Source: CAD feature listing. Evaluate the final solid. Frame: model axes, mm. A direction names the side the tool comes from. Round coordinates to 2 decimals unless told otherwise and drop trailing zeros. Write each loop counter-clockwise with the first axis right and the second up, starting at its lowest first coordinate (ties: lowest second). Pieces come first, ordered by that corner, then holes.
from build123d import *

# Parameters (mm, degrees)
SKETCH1_W          = 98.9
SKETCH1_H          = 124.45
BODY_DEPTH         = 22.55
SKETCH4_W          = 7
SKETCH4_H          = 3
SKETCH4_W_2        = 3
SKETCH4_H_2        = 7
CUT_EXTRUDE1_DEPTH = 63
SKETCH5_W          = 8.299397568
SKETCH5_H          = 10.9
CUT_EXTRUDE2_DEPTH = 63
SKETCH6_W          = 98.9
SKETCH6_H          = 68.5
CUT_EXTRUDE3_DEPTH = 63
SKETCH7_W          = 22.55
SKETCH7_H          = 1.441759006
CUT_EXTRUDE4_DEPTH = 63
SKETCH8_W          = 35
SKETCH8_H          = 13.1
CUT_EXTRUDE5_DEPTH = 23.55
SKETCH9_R          = 1.25
CUT_EXTRUDE6_DEPTH = 10
SKETCH10_R         = 1.25
CUT_EXTRUDE7_DEPTH = 5
CIRPATTERN1_COUNT  = 4


with BuildPart() as part:
    # Sketch1 → body (new body)
    with BuildSketch(Plane.XY):
        Rectangle(SKETCH1_W, SKETCH1_H)
    extrude(amount=BODY_DEPTH)

    # Sketch4 → Cut-Extrude1 (cut)
    with BuildSketch(Plane(origin=(0, 0, 0), x_dir=(-1, 0, 0), z_dir=(0, 0, -1))):
        with Locations((0, 62.225)):
            Rectangle(SKETCH4_W, SKETCH4_H)
        with Locations((49.35, 12.775)):
            Rectangle(SKETCH4_W_2, SKETCH4_H_2)
        with Locations((-49.45, 12.875)):
            Rectangle(SKETCH4_W_2, SKETCH4_H_2)
    extrude(amount=-CUT_EXTRUDE1_DEPTH, mode=Mode.SUBTRACT)

    # Sketch5 → Cut-Extrude2 (cut)
    with BuildSketch(Plane(origin=(0, 0, 0), x_dir=(-1, 0, 0), z_dir=(0, 0, -1))):
        with Locations((-0.05, 12.825)):
            Rectangle(SKETCH5_W, SKETCH5_H)
        with BuildLine():
            Line((4.099698784, 18.275), (4.099698784, 7.375))
            ThreePointArc((4.099698784, 7.375), (6.087912376, 9.783860137), (6.8, 12.825))
            ThreePointArc((6.8, 12.825), (6.087912376, 15.866139863), (4.099698784, 18.275))
        make_face()
        with BuildLine():
            ThreePointArc((-4.199698784, 18.275), (-6.9, 12.825), (-4.199698784, 7.375))
            Line((-4.199698784, 7.375), (-4.199698784, 18.275))
        make_face()
    extrude(amount=-CUT_EXTRUDE2_DEPTH, mode=Mode.SUBTRACT)

    # Sketch6 → Cut-Extrude3 (cut)
    with BuildSketch(Plane(origin=(0, 0, 0), x_dir=(-1, 0, 0), z_dir=(0, 0, -1))):
        with BuildLine():
            Line((49.45, 19.275), (49.45, 62.225))
            Line((49.45, 62.225), (6.5, 62.225))
            Line((6.5, 62.225), (6.5, 22.275))
            ThreePointArc((6.5, 22.275), (8.621320344, 21.396320344), (9.5, 19.275))
            Line((9.5, 19.275), (49.45, 19.275))
        make_face()
        with BuildLine():
            Line((-49.45, 60.783244994), (-49.45, 19.391375139))
            Line((-49.45, 19.391375139), (-9.597617792, 19.297494249))
            ThreePointArc((-9.597617792, 19.297494249), (-8.71394336, 21.416738793), (-6.590558988, 22.290418797))
            Line((-6.590558988, 22.290418797), (-6.496484462, 62.225))
            Line((-6.496484462, 62.225), (-49.446603635, 62.225))
            Line((-49.446603635, 62.225), (-49.45, 60.783244994))
        make_face()
        with Locations((0, -27.975)):
            Rectangle(SKETCH6_W, SKETCH6_H)
    extrude(amount=-CUT_EXTRUDE3_DEPTH, mode=Mode.SUBTRACT)

    # Sketch7 → Cut-Extrude4 (cut)
    with BuildSketch(Plane(origin=(49.592912844, 0.116826812, 0), x_dir=(0, 0, 1), z_dir=(-0.999997225, -0.002355709, 0))):
        with Locations((11.275, 61.387466016)):
            Rectangle(SKETCH7_W, SKETCH7_H)
    extrude(amount=-CUT_EXTRUDE4_DEPTH, mode=Mode.SUBTRACT)

    # Sketch8 → Cut-Extrude5 (cut, through all)
    with BuildSketch(Plane.XY.offset(22.55)):
        with Locations((0, 6.275)):
            Rectangle(SKETCH8_W, SKETCH8_H)
    extrude(amount=-CUT_EXTRUDE5_DEPTH, mode=Mode.SUBTRACT)

    # Sketch9 → Cut-Extrude6 (cut)
    with BuildSketch(Plane.XZ.offset(-12.825)):
        with Locations((13, 11.275)):
            Circle(SKETCH9_R)
        with Locations((-13, 11.275)):
            Circle(SKETCH9_R)
    extrude(amount=-CUT_EXTRUDE6_DEPTH, mode=Mode.SUBTRACT)

    # Sketch10 → Cut-Extrude7 (cut)
    with BuildSketch(Plane(origin=(47.95, 0, 0), x_dir=(0, 0, -1), z_dir=(1, 0, 0))):
        with Locations((-20.05, 12.875)):
            Circle(SKETCH10_R)
        with Locations((-5.05, 12.875)):
            Circle(SKETCH10_R)
    cut_extrude7 = extrude(amount=-CUT_EXTRUDE7_DEPTH, mode=Mode.SUBTRACT)

    # CirPattern1: Cut-Extrude7 ×4 about axis
    cirpattern1_axis = Axis((0.05, 12.825, 0), (0, 0, 1))
    for i in range(1, CIRPATTERN1_COUNT):
        add(cut_extrude7.rotate(cirpattern1_axis, i * 360 / CIRPATTERN1_COUNT), mode=Mode.SUBTRACT)


solid = part.part
1) Section query A-A on x = -13. Return the cut outline in (y, z) (3 decimals), then the cut area to 3 significant figures.
Taken from the geometry:
outline: (12.825, 0) - (19.275, 0) - (19.275, 10.025) - (12.825, 10.025) - close; (12.825, 12.525) - (19.275, 12.525) - (19.275, 22.55) - (12.825, 22.55) - close
area: 129 mm2
2) Contact query for flat-ended pins moving along their axis: P1, Ø2, axis at x = 0, z = 20.05, coming from the +Y side (3 decimals); P2, Ø4, axis at x = 13, z = 11.275, coming from the +Y side; P3, Ø5.5, axis at y = 14.5, z = 12, coming from the -X side; P4, Ø4, axis at x = -1.5, z = 11.5, coming from the -Y side (3 decimals). Output: stop coordinate, or through.
Taken from the geometry:
P1: stops at y = 55.725
P2: stops at y = 19.31
P3: stops at x = -49.45
P4: stops at y = 18.275
3) Material intervals for line 1 (Y direction, x = 44.4, z = 5.05) (3 decimals); line 2 (Y direction, x = -46.1, z = 20.05) (3 decimals); line 3 (Y direction, x = 4, z = 3) (3 decimals), sorted ascending.
Taken from the geometry:
line 1: y = 6.275 to 11.625, 14.125 to 19.379
line 2: y = 6.275 to 11.525, 14.025 to 19.275
line 3: y = 18.275 to 62.225
4) Pull-direction query (X, two-part tool) for faces 5 (the face through (-5, 62.225, 11)), 6 (the face through (0, 18.275, 11)), 7 (the face through (12.729, 16.021, 10.055)), 8 (the face through (49.45, 8, 11)); classes: released by +X, released by -X, zero draft, split by the parting line, or undercut.
Taken from the geometry:
face 5: zero draft
face 6: undercut
face 7: undercut
face 8: released by +X
5) Section query C-C on x = 0. Return the cut outline in (y, z) (3 decimals).
Taken from the geometry:
outline: (18.275, 0) - (60.725, 0) - (60.725, 3.8) - (55.725, 3.8) - (55.725, 6.3) - (60.725, 6.3) - (60.725, 18.8) - (55.725, 18.8) - (55.725, 21.3) - (60.725, 21.3) - (60.725, 22.55) - (18.275, 22.55) - close
6) Reachability of faces 1 (the face through (-17.5, 10, 11)), 2 (the face through (0.479, 58.26, 18.895)), 3 (the face through (-42.85, 13, 5)), 4 (the face through (-29, 19.275, 11)) from +Z, -Z, +X, -X, +Y, -Y: full face, straight path, thin tool, end or side. Return the list, or none.
Taken from the geometry:
face 1: +Z, -Z, -Y
face 2: +Y
face 3: -X
face 4: +Z, -Z, -X, +Y
7) Section query D-D on y = 58.5. Return the cut outline in (x, z), then the cut area to 3 significant figures.
Taken from the geometry:
outline: (-6.5, 0) - (6.51, 0) - (6.51, 22.55) - (-6.5, 22.55) - close; hole circle Ø2.5 at (0, 5.05); hole circle Ø2.5 at (0, 20.05)
area: 283 mm2
